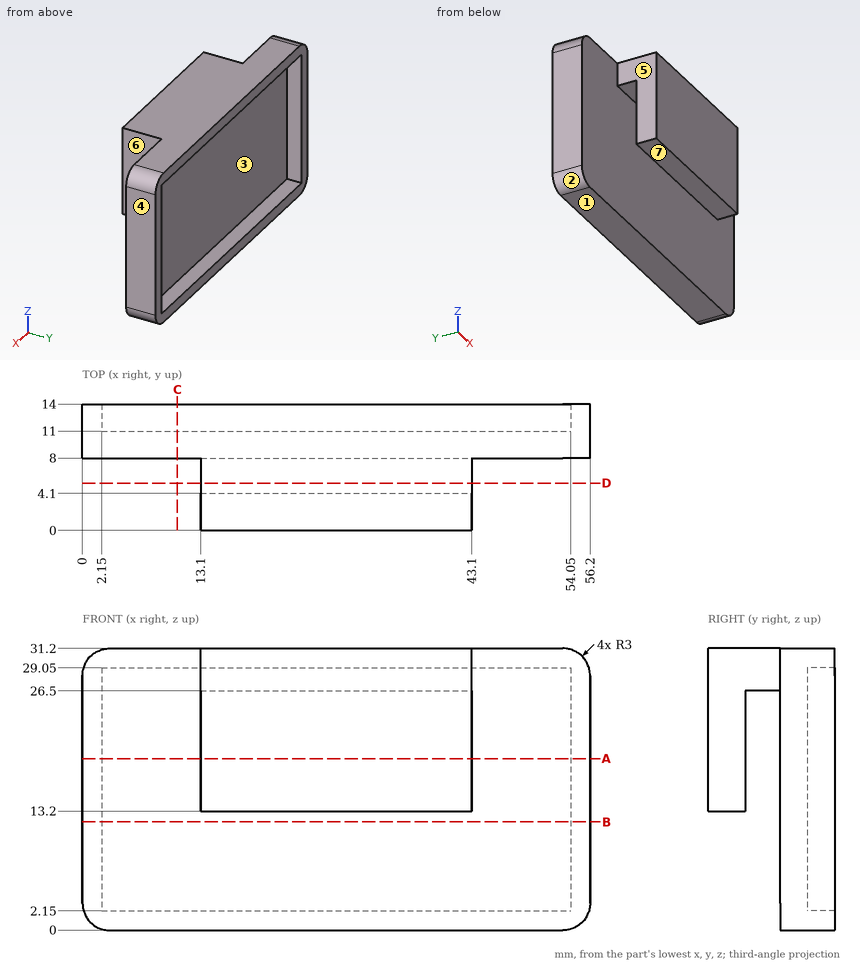
Here's the drawing with two shaded views (mm, measured from the low corner). I have some questions. A direction names the side the tool comes from. Round coordinates to 2 decimals unless told otherwise and drop trailing zeros. Order: outer loops, then holes, each group sorted by start corner. A loop starts at its lowest first (then second) coordinate and runs counter-clockwise, first axis right, second up. Notation, with made-up numbers: M 40.5,61.25 L 88.5,61.25 A15 ccw 88.5,69.25 Z; hole C -1.5,33 d6. An arc over 180 degrees is marked long. Use CSV: the item, a comma, the result in double quotes.
1) I want a section at B-B (z = 12). List the corners of the cut face in (x, y) for me.
Taken from the geometry:
outline,"M 0,8 L 56.2,8 L 56.2,14 L 54.05,14 L 54.05,11 L 2.15,11 L 2.15,14 L 0,14 Z"
2) On a 3-axis mill with a long thin cutter (end or side, diameter ignored), from which of +Z, -Z, +X, -X, +Y, -Y can I reach the whole of each face in a straight line? I mean the marked faces 5, 6 and 7. Say none if no direction works.
Taken from the geometry:
face 5,"+Z, -Z, -X, -Y"
face 6,"+Z, -Z, +X, -Y"
face 7,"-Z, +X, -X, -Y"
3) I want a section at A-A (z = 19). List the corners of the cut face in (x, y) for me.
Taken from the geometry:
outline,"M 0,8 L 56.2,8 L 56.2,14 L 54.05,14 L 54.05,11 L 2.15,11 L 2.15,14 L 0,14 Z; M 13.1,0 L 43.1,0 L 43.1,4.1 L 13.1,4.1 Z"
4) I need wall thicknesses on line 1 along X through (y, z) = (12.75, 25); line 2 along Y through (x, z) = (39, 25); line 3 along Y through (x, z) = (24.5, 28.5). Which ranges of each line are inside material? Lowest first, please. Write a range as [from, to].
Taken from the geometry:
line 1,"[0, 2.15], [54.05, 56.2]"
line 2,"[0, 4.1], [8, 11]"
line 3,"[0, 11]"
5) I'm going to push flat-ended pins straight in: P1, Ø0.9, axis at x = 32.5, y = 13, coming from the -Z side; P2, Ø6.5, axis at x = 31.5, z = 19.5, coming from the +Y side; P3, Ø1, axis at x = 21.5, y = 4, coming from the -Z side; P4, Ø4, axis at y = 3.5, z = 20, coming from the +X side. Where does each tip first touch, or does it pass through?
Taken from the geometry:
P1,"z = 0"
P2,"y = 11"
P3,"z = 13.2"
P4,"x = 43.1"
6) I want a section at C-C (x = 10.5). List the corners of the cut face in (y, z) for me.
Taken from the geometry:
outline,"M 8,0 L 14,0 L 14,2.15 L 11,2.15 L 11,29.05 L 14,29.05 L 14,31.2 L 8,31.2 Z"
7) If we mould it in two halves opening along X, with no side actions, what happens to the marked faces 1, 2, 3 and 4? For each: pulls with the +X half, pulls with the -X half, needs draft (parallel to the pull), parting line crosses it, or undercut.
Taken from the geometry:
face 1,"needs draft"
face 2,"pulls with the -X half"
face 3,"undercut"
face 4,"pulls with the +X half"
8) I want a section at D-D (y = 5.25). List the corners of the cut face in (x, z) for me.
Taken from the geometry:
outline,"M 13.1,26.5 L 43.1,26.5 L 43.1,31.2 L 13.1,31.2 Z"
